Design review of the part built by this model. Coordinates are the model's own, in mm. A direction names the side the tool comes from. Give positions to 0.01 mm unless a question says otherwise; leave off trailing zeros. Loops run counter-clockwise (first coordinate to the right, second up) from the corner with the lowest first, then second, coordinate; pieces in that order, holes last. Notation, with made-up numbers: (14.5, -7.5) -> (58.5, -7.5) arc R14 cw to (58.5, 14.5) -> close; hole circle Ø1 at (3, -25.75). An arc over 180 degrees is marked (long way). Use a Markdown table: item, result. Add a question column.
1. Add section C-C (y = 27.15). State the section outline as (x, z) points.
2. Add section A-A (y = 0). Count the separate pieces of the cut face and the enclosed holes in it, and give its area (3 significant figures).
3. To check wall thickness, follow line 1 (Y direction, x = 4.5, z = 2); line 2 (Z direction, x = 1, y = -13); line 3 (Z direction, x = 1.5, y = -4). State the ranges of each line that lie inside material, in increasing order.
4. Draft analysis for pull direction Z (two halves, no side actions). For faces 6 (the cylindrical face through (3.3, 17.85, -15.89)), 7 (the flat face through (-8.5, 5, 17)), 8 (the flat face through (2.6, -9.6, 14.3)), state which applies: pulls with the +Z half, pulls with the -Z half, needs draft (parallel to the pull), parting line crosses it, or undercut.
5. Add section D-D (z = -12). State the section outline as (x, y) points.
6. For pin 1 Ø1 at (x, y) = (-1, -5.5) entering from -Z; pin 2 Ø1.8 at (x, y) = (4, 28) entering from +Z; pin 3 Ø2.5 at (y, z) = (4, 16.5) entering from +X, all flat-tipped, find the tip position at first contact; note any pin that passes through.
7. Add section B-B (z = 2.5). State the section outline as (x, y) points, and give its area (3 significant figures).
8. For faces 1 (the flat face through (-2, -8.85, 17)), 2 (the flat face through (5, 25, -6.45)), 3 (the flat face through (3, 3, -14.408)), 4 (the flat face through (-1, 18.15, 17)), 5 (the flat face through (-4, 4, 13.55)), list the 3-axis set-ups (+Z, -Z, +X, -X, +Y, -Y) from which the entire face can be reached by the end or side of a thin tool; tool diameter is ignored.
```python
from build123d import *

# Parameters (mm, degrees)
SKETCH_1_W               = 27.1
SKETCH_1_H               = 42.3
SKETCH_1_W_2             = 21.1
SKETCH_1_H_2             = 36.3
EXTRUDE_1_DEPTH          = 6.5
CHAMFER_1_SIZE           = 3
EXTRUDE_2_DEPTH          = 8.7
EXTRUDE_2_DEPTH_BACK     = 6.5
SKETCH_2_W               = 5
SKETCH_2_H               = 24.3
SKETCH_2_R               = 1.475
SKETCH_3_W               = 27.1
SKETCH_3_H               = 15
EXTRUDE_3_DEPTH          = 6.5
SKETCH_4_W               = 17.60784849
SKETCH_4_H               = 15
EXTRUDE_4_DEPTH          = 6.5
SKETCH_5_W               = 20
SKETCH_5_H               = 11
SKETCH_5_W_2             = 5
SKETCH_5_H_2             = 36.3
EXTRUDE_5_DEPTH          = 6.5
CUT_EXTRUDE_5_DEPTH      = 47.31872216
CUT_EXTRUDE_5_DEPTH_BACK = 47.31872216
SKETCH_6_W               = 20
SKETCH_6_H               = 11.2
CUT_EXTRUDE_6_DEPTH      = 48.966384297
CUT_EXTRUDE_6_DEPTH_BACK = 48.966384297
SKETCH_9_W               = 5
SKETCH_9_H               = 24.3
SKETCH_10_W              = 20
SKETCH_10_H              = 11.2
EXTRUDE_6_DEPTH          = 3
CUT_EXTRUDE_7_DEPTH      = 46.956327339
CUT_EXTRUDE_7_DEPTH_BACK = 46.956327339
SKETCH_11_W              = 13
SKETCH_11_H              = 15
EXTRUDE_7_DEPTH          = 8.5
EXTRUDE_7_DEPTH_BACK     = 5
SKETCH_13_W              = 6
SKETCH_13_H              = 27
CHAMFER_2_SIZE           = 1.5
SKETCH_14_W              = 16.26
SKETCH_14_H              = 36.46
SKETCH_14_W_2            = 16.1
SKETCH_14_H_2            = 36.3
CUT_EXTRUDE_8_DEPTH      = 40.412878606
SKETCH_15_W              = 7.60784849
SKETCH_15_H              = 39.3
EXTRUDE_8_DEPTH          = 6
CUT_EXTRUDE_9_DEPTH      = 6
EXTRUDE_9_DEPTH          = 0.5
CUT_EXTRUDE_10_DEPTH     = 40.412878606
CUT_EXTRUDE_11_DEPTH     = 10


with BuildPart() as part:
    # 草图1 → 凸台-拉伸1 (new body)
    with BuildSketch(Plane(origin=(0, 0, 0), x_dir=(0, 0, -1), z_dir=(1, 0, 0))):
        Rectangle(SKETCH_1_W, SKETCH_1_H)
        Rectangle(SKETCH_1_W_2, SKETCH_1_H_2, mode=Mode.SUBTRACT)
    extrude(amount=EXTRUDE_1_DEPTH)

    # 倒角1
    chamfer_1_edges = [part.edges().sort_by_distance(p)[0] for p in [
        (3.25, 21.15, 13.55),
        (3.25, 21.15, -13.55),
        (3.25, -21.15, -13.55),
        (3.25, -21.15, 13.55),
    ]]
    chamfer(chamfer_1_edges, length=CHAMFER_1_SIZE)

    # 草图2 → 凸台-拉伸2 (add, two sides: drawn at the far end of the back side and taken through both)
    with BuildSketch(Plane.ZY.offset(-EXTRUDE_2_DEPTH_BACK)):
        with Locations((16.05, 0)):
            Rectangle(SKETCH_2_W, SKETCH_2_H)
        with Locations((16.05, 7.15)):
            Circle(SKETCH_2_R, mode=Mode.SUBTRACT)
        with Locations((16.05, -7.15)):
            Circle(SKETCH_2_R, mode=Mode.SUBTRACT)
    extrude(amount=EXTRUDE_2_DEPTH + EXTRUDE_2_DEPTH_BACK)

    # 草图3 → 凸台-拉伸3 (add)
    with BuildSketch(Plane(origin=(6.5, 0, 0), x_dir=(0, 0, -1), z_dir=(1, 0, 0))):
        with Locations((0, 25.65)):
            Rectangle(SKETCH_3_W, SKETCH_3_H)
    extrude(amount=-EXTRUDE_3_DEPTH)

    # 草图4 → 凸台-拉伸4 (add)
    with BuildSketch(Plane.ZY):
        with Locations((-22.353924245, 25.65)):
            Rectangle(SKETCH_4_W, SKETCH_4_H)
    extrude(amount=-EXTRUDE_4_DEPTH)

    # 草图5 → 凸台-拉伸5 (add)
    with BuildSketch(Plane.ZY):
        with Locations((3.55, 25.714062057)):
            Rectangle(SKETCH_5_W, SKETCH_5_H)
        with Locations((-8.05, 0)):
            Rectangle(SKETCH_5_W_2, SKETCH_5_H_2)
    extrude(amount=-EXTRUDE_5_DEPTH)

    # 草图6 → 切除-拉伸5 (cut, two sides: drawn at the far end of the back side and taken through both)
    with BuildSketch(Plane.ZY.offset(-CUT_EXTRUDE_5_DEPTH_BACK)):
        with Locations((3.55, 25.55)):
            Rectangle(SKETCH_6_W, SKETCH_6_H)
    extrude(amount=CUT_EXTRUDE_5_DEPTH + CUT_EXTRUDE_5_DEPTH_BACK, mode=Mode.SUBTRACT)

    # 草图9 → 切除-拉伸6 (cut, two sides: drawn at the far end of the back side and taken through both)
    with BuildSketch(Plane.ZY.offset(8.7).offset(-CUT_EXTRUDE_6_DEPTH_BACK)):
        with Locations((16.05, 0)):
            Rectangle(SKETCH_9_W, SKETCH_9_H)
    extrude(amount=CUT_EXTRUDE_6_DEPTH + CUT_EXTRUDE_6_DEPTH_BACK, mode=Mode.SUBTRACT)

    # 草图10 → 凸台-拉伸6 (add)
    with BuildSketch(Plane.ZY):
        with Locations((3.55, 25.55)):
            Rectangle(SKETCH_10_W, SKETCH_10_H)
    extrude(amount=-EXTRUDE_6_DEPTH)

    # 草图11 → 切除-拉伸7 (cut, two sides: drawn at the far end of the back side and taken through both)
    with BuildSketch(Plane(origin=(6.5, 0, 0), x_dir=(0, 0, -1), z_dir=(1, 0, 0)).offset(-CUT_EXTRUDE_7_DEPTH_BACK)):
        with Locations((24.65784849, 25.65)):
            Rectangle(SKETCH_11_W, SKETCH_11_H)
    extrude(amount=CUT_EXTRUDE_7_DEPTH + CUT_EXTRUDE_7_DEPTH_BACK, mode=Mode.SUBTRACT)

    # 草图13 → 凸台-拉伸7 (add, two sides: drawn at the far end of the back side and taken through both)
    with BuildSketch(Plane.ZY.offset(-EXTRUDE_7_DEPTH_BACK)):
        with Locations((16.55, 4.65)):
            Rectangle(SKETCH_13_W, SKETCH_13_H)
    extrude(amount=EXTRUDE_7_DEPTH + EXTRUDE_7_DEPTH_BACK)

    # 倒角2
    chamfer_2_edges = [part.edges().sort_by_distance(p)[0] for p in [
        (5, 4.65, 13.55),
        (2.5, -8.85, 13.55),
    ]]
    chamfer(chamfer_2_edges, length=CHAMFER_2_SIZE - 0.0001)  # a hair under: the kernel refuses the full size

    # 草图14 → 切除-拉伸8 (cut, through all)
    with BuildSketch(Plane.ZY):
        with Locations((2.5, 0)):
            Rectangle(SKETCH_14_W, SKETCH_14_H)
        with Locations((2.5, 0)):
            Rectangle(SKETCH_14_W_2, SKETCH_14_H_2, mode=Mode.SUBTRACT)
    extrude(amount=-CUT_EXTRUDE_8_DEPTH, mode=Mode.SUBTRACT)

    # 草图15 → 凸台-拉伸8 (add)
    with BuildSketch(Plane(origin=(6.5, 0, 0), x_dir=(0, 0, -1), z_dir=(1, 0, 0))):
        with Locations((14.353924245, -1.5)):
            Rectangle(SKETCH_15_W, SKETCH_15_H)
    extrude(amount=-EXTRUDE_8_DEPTH)

    # 草图16 → 切除-拉伸9 (cut)
    with BuildSketch(Plane(origin=(3, 0, 0), x_dir=(0, 0, -1), z_dir=(1, 0, 0))):
        with BuildLine():
            Line((-8.55, 28.65), (1.45, 28.65))
            ThreePointArc((1.45, 28.65), (2.95, 27.15), (1.45, 25.65))
            Line((1.45, 25.65), (-8.55, 25.65))
            ThreePointArc((-8.55, 25.65), (-10.05, 27.15), (-8.55, 28.65))
        make_face()
    extrude(amount=-CUT_EXTRUDE_9_DEPTH, mode=Mode.SUBTRACT)

    # 草图17 → 凸台-拉伸9 (add)
    with BuildSketch(Plane.ZY.offset(-0.5)):
        Polygon((-13.55, -18.15), (-13.55, 18.15), (-18.15784849, 18.15), (-18.15784849, -21.15), (-10.55, -21.15), align=None)
    extrude(amount=EXTRUDE_9_DEPTH)

    # 草图18 → 切除-拉伸10 (cut, through all)
    with BuildSketch(Plane.ZY):
        with BuildLine():
            Line((-14.40784849, 11.85), (-14.40784849, -11.15))
            ThreePointArc((-14.40784849, -11.15), (-15.85784849, -12.6), (-17.30784849, -11.15))
            Line((-17.30784849, -11.15), (-17.30784849, 11.85))
            ThreePointArc((-17.30784849, 11.85), (-15.85784849, 13.3), (-14.40784849, 11.85))
        make_face()
    extrude(amount=-CUT_EXTRUDE_10_DEPTH, mode=Mode.SUBTRACT)

    # 草图19 → 切除-拉伸11 (cut)
    with BuildSketch(Plane(origin=(6.5, 0, 0), x_dir=(0, 0, -1), z_dir=(1, 0, 0))):
        with BuildLine():
            Line((14.40784849, 11.85), (17.30784849, 11.85))
            Line((17.30784849, 11.85), (17.30784849, 16.4))
            ThreePointArc((17.30784849, 16.4), (15.85784849, 17.85), (14.40784849, 16.4))
            Line((14.40784849, 16.4), (14.40784849, 11.85))
        make_face()
    extrude(amount=-CUT_EXTRUDE_11_DEPTH, mode=Mode.SUBTRACT)


solid = part.part
```
Taken from the geometry:
| question | item | result |
|---|---|---|
| 1 | outline | (0, -18.16) -> (6.5, -18.16) -> (6.5, -6.45) -> (3, -6.45) -> (3, -2.95) -> (0, -2.95) -> close; (0, 10.05) -> (3, 10.05) -> (3, 13.55) -> (0, 13.55) -> close |
| 2 | separate pieces | 3 |
| 2 | enclosed holes | 0 |
| 2 | area | 164 mm^2 |
| 3 | line 1 | y = -21.15 to -18.23, 18.23 to 19.95, 31.15 to 33.15 |
| 3 | line 2 | z = -18.16 to -5.63, 10.63 to 13.55 |
| 3 | line 3 | z = -18.16 to -17.31, -14.41 to -5.63, 10.63 to 19.55 |
| 4 | face 6 | undercut |
| 4 | face 7 | needs draft |
| 4 | face 8 | pulls with the +Z half |
| 5 | outline | (0, -21.15) -> (6.5, -21.15) -> (6.5, 33.15) -> (0, 33.15) -> close |
| 6 | pin 1 | stops at z = 13.55 |
| 6 | pin 2 | stops at z = -6.45 |
| 6 | pin 3 | stops at x = 5 |
| 7 | outline | (0, -21.15) -> (6.5, -21.15) -> (6.5, -18.23) -> (0, -18.23) -> close; (0, 18.23) -> (6.5, 18.23) -> (6.5, 19.95) -> (3, 19.95) -> (3, 25.65) -> (0, 25.65) -> close; (0, 28.65) -> (3, 28.65) -> (3, 31.15) -> (6.5, 31.15) -> (6.5, 33.15) -> (0, 33.15) -> close |
| 7 | area | 67.8 mm^2 |
| 8 | face 1 | +Z, -X, -Y |
| 8 | face 2 | +Z, +X |
| 8 | face 3 | +X, -X |
| 8 | face 4 | +Z, +X, -X, +Y |
| 8 | face 5 | -Z, -X, +Y, -Y |
